Verification items for the finished model (mm, model axes). Face numbers are marked on the shaded views. A direction names the side the tool comes from. Coordinates: 2 decimals unless noted, no trailing zeros. Loops run counter-clockwise (first coordinate to the right, second up) from the corner with the lowest first, then second, coordinate; pieces in that order, holes last. Notation, with made-up numbers: (21, 59) - (46, 59) arc R29 ccw to (46, 92) - close; hole circle Ø7 at (86, 24.5). An arc over 180 degrees is marked (long way). Answer as CSV lines item,"result". Start each with the question number.
1. Set-up check for the marked faces 4 and 5: record each of +Z, -Z, +X, -X, +Y, -Y from which the full face is reachable in a straight line by a thin tool's end or side.
2. Gauge pin test, flat ends, axial feed: P1, Ø6.5, axis at x = 20, z = 6, coming from the +Y side; P2, Ø24, axis at y = 24, z = 6.5, coming from the +X side; P3, Ø2, axis at y = 9.5, z = -19.5, coming from the +X side. Record the tip position at first contact, or that the pin passes through.
3. Cross-section at B-B (z = 20). Enter the section's corners in (x, y).
4. Release check for a two-part mould opening along X. For the marked faces 1, 2 and 3 record: pulls with the +X half, pulls with the -X half, needs draft (parallel to the pull), parting line crosses it, or undercut.
5. Material ranges on line 1 (Z direction, x = 20, y = 3); line 2 (X direction, y = 24, z = -16.5), recorded low to high. Write a range as [from, to].
6. Cross-section at A-A (y = 20). Enter the section's corners in (x, z), plus the area to 3 significant figures.
7. Cross-section at D-D (y = 30.5). Enter the section's corners in (x, z), plus the area to 3 significant figures.
```python
from build123d import *

# Parameters (mm, degrees)
BOSS_EXTRUDE1_DEPTH = 38
SKETCH2_R           = 4.5
CUT_EXTRUDE1_DEPTH  = 41
SKETCH3_R           = 4.5
CUT_EXTRUDE2_DEPTH  = 41


with BuildPart() as part:
    # Sketch1 → Boss-Extrude1 (new body, symmetric)
    with BuildSketch(Plane.XY):
        with BuildLine():
            Line((0, 0), (0, 40))
            ThreePointArc((0, 40), (4.242640687, 38.242640687), (6, 34))
            Line((6, 34), (6, 12))
            ThreePointArc((6, 12), (7.757359313, 7.757359313), (12, 6))
            Line((12, 6), (34, 6))
            ThreePointArc((34, 6), (38.242640687, 4.242640687), (40, 0))
            Line((40, 0), (0, 0))
        make_face()
    extrude(amount=BOSS_EXTRUDE1_DEPTH, both=True)

    # Sketch2 → Cut-Extrude1 (cut, through all)
    with BuildSketch(Plane(origin=(0, 0, 0), x_dir=(1, 0, 0), z_dir=(0, 1, 0))):
        with Locations((20, -20)):
            Circle(SKETCH2_R)
        with Locations((20, 20)):
            Circle(SKETCH2_R)
    extrude(amount=CUT_EXTRUDE1_DEPTH, mode=Mode.SUBTRACT)

    # Sketch3 → Cut-Extrude2 (cut, through all)
    with BuildSketch(Plane(origin=(0, 0, 0), x_dir=(0, 0, -1), z_dir=(1, 0, 0))):
        with Locations((-20, 20)):
            Circle(SKETCH3_R)
        with Locations((20, 20)):
            Circle(SKETCH3_R)
    extrude(amount=CUT_EXTRUDE2_DEPTH, mode=Mode.SUBTRACT)


solid = part.part
```
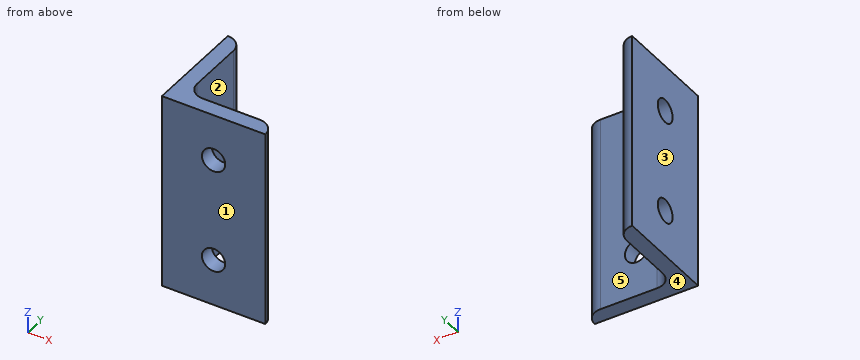
Values follow:
1,face 4,"-Z, +X, -X, +Y, -Y"
1,face 5,"+Z, -Z, +X, +Y"
2,P1,"stops at y = 6"
2,P2,"stops at x = 6"
2,P3,"stops at x = 7.13"
3,outline,"(0, 0) - (15.5, 0) - (15.5, 6) - (12, 6) arc R6 cw to (6, 12) - (6, 15.5) - (0, 15.5) - close; (0, 24.5) - (6, 24.5) - (6, 34) arc R6 ccw to (0, 40) - close; (24.5, 0) - (40, 0) arc R6 ccw to (34, 6) - (24.5, 6) - close"
4,face 1,"needs draft"
4,face 2,"pulls with the +X half"
4,face 3,"pulls with the -X half"
5,line 1,"z = [-38, -24.5], [-15.5, 15.5], [24.5, 38]"
5,line 2,"x = [0, 6]"
6,outline,"(0, -38) - (6, -38) - (6, -24.5) - (0, -24.5) - close; (0, -15.5) - (6, -15.5) - (6, 15.5) - (0, 15.5) - close; (0, 24.5) - (6, 24.5) - (6, 38) - (0, 38) - close"
6,area,"348 mm²"
7,outline,"(0, -38) - (6, -38) - (6, 38) - (0, 38) - close"
7,area,"456 mm²"
